The listing builds one solid part. Answer for the finished solid, in the listing's coordinates (mm). A direction names the side the tool comes from. Give positions to 0.01 mm unless a question says otherwise; leave off trailing zeros. Order: outer loops, then holes, each group sorted by start corner. A loop starts at its lowest first (then second) coordinate and runs counter-clockwise, first axis right, second up.
```python
from build123d import *

# Parameters (mm, degrees)
SKETCH2_W                       = 38.1
SKETCH2_H                       = 38.1
BOSS_EXTRUDE1_DEPTH             = 6.35
BOSS_EXTRUDE2_DEPTH             = 156.456983
SKETCH4_W                       = 38.1
SKETCH4_H                       = 38.1
BOSS_EXTRUDE3_DEPTH             = 6.35
FILLET1_R                       = 3.175
F_1_4_0_25_DIAMETER_HOLE1_D     = 6.35
F_1_4_0_25_DIAMETER_HOLE1_DEPTH = 25.603542527
CUT_EXTRUDE1_REACH              = 187.255
LPATTERN1_COUNT                 = 4
LPATTERN1_PITCH                 = 38.1


with BuildPart() as part:
    # Sketch2 → Boss-Extrude1 (new body)
    with BuildSketch(Plane(origin=(0, 0, 0), x_dir=(0.1994825347085473, 0.06819943394704729, 0.9775252199076787), z_dir=(-0.924962461700774, -0.31622776601683794, 0.21081851067789195))):
        Rectangle(SKETCH2_W, SKETCH2_H)
    extrude(amount=BOSS_EXTRUDE1_DEPTH)

    # Sketch3 → Boss-Extrude2 (add)
    with BuildSketch(Plane(origin=(-5.873511632, -2.008046314, 1.338697543), x_dir=(0.19948253470854727, 0.06819943394704733, 0.9775252199076787), z_dir=(-0.9249624617007739, -0.316227766016838, 0.21081851067789192))):
        Polygon((-15.875, -15.875), (0, -15.875), (0, -19.05), (-19.05, -19.05), (-19.05, 19.05), (0, 19.05), (0, 15.875), (-15.875, 15.875), align=None)
    extrude(amount=BOSS_EXTRUDE2_DEPTH)

    # Sketch4 → Boss-Extrude3 (add)
    with BuildSketch(Plane(origin=(-150.590347718, -51.484088506, 34.32272567), x_dir=(0.19948253470854724, 0.06819943394704728, 0.9775252199076787), z_dir=(-0.924962461700774, -0.31622776601683794, 0.2108185106778919))):
        Rectangle(SKETCH4_W, SKETCH4_H)
    extrude(amount=-BOSS_EXTRUDE3_DEPTH)

    # Fillet1
    fillet1_edges = [part.edges().sort_by_distance(p)[0] for p in [
        (-2.321368427, -17.570760643, -6.42040889),
        (-12.592440075, 12.472002, -6.42040889),
        (-141.164692882, -65.03875652, 25.224921695),
        (-151.435764529, -34.995993877, 25.224921695),
    ]]
    fillet(fillet1_edges, radius=FILLET1_R)

    # 1/4 (0.25) Diameter Hole1
    with Locations(Plane(origin=(-144.716836086, -49.476042191, 32.984028128), x_dir=(-0.19948253470854763, -0.06819943394704747, -0.9775252199076786), z_dir=(0.924962461700774, 0.3162277660168374, -0.2108185106778923))):
        with Locations((9.525, -6.35), (-12.7, -12.7), (-12.7, 12.7), (9.47011661, 6.35)):
            f_1_4_0_25_diameter_hole1 = Hole(F_1_4_0_25_DIAMETER_HOLE1_D / 2, depth=F_1_4_0_25_DIAMETER_HOLE1_DEPTH)

    # Mirror1: 1/4 (0.25) Diameter Hole1 across plane
    add(f_1_4_0_25_diameter_hole1.mirror(Plane(origin=(-75.295173859, -25.742044253, 17.161362835), x_dir=(0.19948253470854732, 0.06819943394704736, 0.9775252199076787), z_dir=(0.924962461700774, 0.316227766016838, -0.21081851067789195))), mode=Mode.SUBTRACT)

    # Sketch9 → Cut-Extrude1 (cut, up to next)
    with BuildSketch(Plane(origin=(-3.166785238, -1.082666014, -15.518212866), x_dir=(0.9799013819493537, -0.013883637884437966, -0.19899880967694392), z_dir=(0.19948253470854727, 0.06819943394704746, 0.9775252199076788)), mode=Mode.PRIVATE) as cut_extrude1_sk1:
        with BuildLine():
            Line((-4.984618665, -11.137455788), (-11.58066581, 7.722289794))
            ThreePointArc((-11.58066581, 7.722289794), (-12.390150485, 8.628384663), (-13.603248415, 8.696698385))
            Line((-13.603248415, 8.696698385), (-32.462993997, 2.100651241))
            ThreePointArc((-32.462993997, 2.100651241), (-33.523895818, 0.691411823), (-32.627917913, -0.828026233))
            Line((-32.627917913, -0.828026233), (-7.172125187, -13.091724671))
            ThreePointArc((-7.172125187, -13.091724671), (-5.425471566, -12.845412794), (-4.984618665, -11.137455788))
        make_face()
    cut_extrude1_tool1 = extrude(cut_extrude1_sk1.sketch, amount=-CUT_EXTRUDE1_REACH, mode=Mode.PRIVATE) & part.part
    # Sketch9 → Cut-Extrude1 (cut, up to next)
    with BuildSketch(Plane(origin=(-3.166785238, -1.082666014, -15.518212866), x_dir=(0.9799013819493537, -0.013883637884437966, -0.19899880967694392), z_dir=(0.19948253470854727, 0.06819943394704746, 0.9775252199076788)), mode=Mode.PRIVATE) as cut_extrude1_sk2:
        with BuildLine():
            Line((-38.621900308, -2.924374261), (-13.166107581, -15.188072699))
            ThreePointArc((-13.166107581, -15.188072699), (-12.270129676, -16.707510755), (-13.331031497, -18.116750174))
            Line((-13.331031497, -18.116750174), (-32.190777079, -24.712797318))
            ThreePointArc((-32.190777079, -24.712797318), (-33.403875009, -24.644483595), (-34.213359685, -23.738388726))
            Line((-34.213359685, -23.738388726), (-40.809406829, -4.878643144))
            ThreePointArc((-40.809406829, -4.878643144), (-40.368553929, -3.170686139), (-38.621900308, -2.924374261))
        make_face()
    cut_extrude1_tool2 = extrude(cut_extrude1_sk2.sketch, amount=-CUT_EXTRUDE1_REACH, mode=Mode.PRIVATE) & part.part
    cut_extrude1_1 = cut_extrude1_tool1.solids().sort_by_distance((-20.084687, -2.329504, -11.978806))[0]
    add(cut_extrude1_1, mode=Mode.SUBTRACT)
    cut_extrude1_2 = cut_extrude1_tool2.solids().sort_by_distance((-31.122512, -15.177301, -8.829971))[0]
    add(cut_extrude1_2, mode=Mode.SUBTRACT)
    cut_extrude1 = cut_extrude1_1 + cut_extrude1_2  # Cut-Extrude1 as one shape, for the pattern or mirror that repeats it

    # LPattern1: Cut-Extrude1 ×4
    with Locations(*[Vector(-0.924962461700774, -0.3162277660168377, 0.210818510677892) * (i * LPATTERN1_PITCH) for i in range(1, LPATTERN1_COUNT)]):
        add(cut_extrude1, mode=Mode.SUBTRACT)


solid = part.part
```
1) Given P1, Ø8, axis at x = -53.5, z = -7, coming from the +Y side; P2, Ø8, axis at x = -70.5, y = -52.5, coming from the -Z side, each flat-ended and moving along its own axis, determine where each tip first touches the part or whether it passes through.
Geometry says:
P1: stops at y = 3.21
P2: passes through
2) A tool of negligible diameter and unlimited length cuts with its end or side. For faces 1 (the flat face through (-82.03, -27.01, 0.78)), 2 (the cylindrical face through (-140.614, -63.841, 25.143)), 3 (the flat face through (-58.39, -19.82, -4.54)), 4 (the flat face through (-96.402, -19.536, 3.194)), from which of +Z, -Z, +X, -X, +Y, -Y can it reach the whole face along a straight path? Write none if from no direction.
Geometry says:
face 1: +Z
face 2: none
face 3: -Z
face 4: +Z, -Z
3) Find section A-A (x = -24.5). Write down the section's boundary in (y, z).
Geometry says:
outline: (-28.51, -12.5) - (-21.8, -12.97) - (-21.8, -9.72) - (-25.15, -9.49) - (-25.15, 6.75) - (-28.51, 6.99) - close; (-12.33, -13.63) - (-7.36, -13.97) - (-6.82, -10.76) - (-11.8, -10.42) - close; (5.05, -14.84) - (11.76, -15.31) - (11.76, 4.18) - (8.4, 4.41) - (8.4, -11.83) - (5.05, -11.59) - close
4) Find section B-B (z = 46). Count the separate pieces of the cut face and the enclosed holes in it, then the cut area to 3 significant figures.
Geometry says:
separate pieces: 3
enclosed holes: 0
area: 166 mm2
5) Straight lines are drawn through the part: probe 1 along Y at (x, z) = (-53.5, -0.5); probe 2 along Y at (x, z) = (-26.5, 6); probe 3 along X at (y, z) = (-49.5, 31). For each, find the intervals that lie inside material, in ascending order.
Geometry says:
probe 1: y = -38.42 to -35.07, -1.51 to 1.84
probe 2: y = -29.19 to -25.84
probe 3: x = -152.03 to -145.16
6) For a pull along X with two mould halves and no side action, classify faces 5 (the cylindrical face through (-121.225, -53.805, 10.651)), 6 (the cylindrical face through (-36.33, -0.01, -10.43)) as +X half, -X half, draft (parallel to the pull), parting line (faces both ways), or undercut.
Geometry says:
face 5: -X half
face 6: undercut
